Build history of the part. All positions in model axes, mm. Face numbers are marked on the shaded views. Round coordinates to 2 decimals unless told otherwise and drop trailing zeros. Order: outer loops, then holes, each group sorted by start corner. A loop starts at its lowest first (then second) coordinate and runs counter-clockwise, first axis right, second up. Notation, with made-up numbers: (76, 6) -> (132, 6) arc R36 cw to (132, 40) -> close; hole circle Ø6 at (72.25, -13). An arc over 180 degrees is marked (long way). Use a Markdown table: item, result. Add a question column.
Item 1: Pin check, flat tips, straight feed: pin 1 (3 mm diameter, centred on x = 10, y = 9, fed in from +Z); pin 2 (1.5 mm diameter, centred on y = 15, z = -1.5, fed in from +X); pin 3 (3 mm diameter, centred on x = 4.5, z = 16.5, fed in from -Y); pin 4 (6 mm diameter, centred on x = 13.5, z = 4, fed in from -Y). Stop position of each tip, or through.
Item 2: Slice it at C-C, the plane z = 8.5. Give the cut face in (x, y), plus the area to 3 significant figures.
Item 3: Probe L1, parallel to Y at x = 0.95, z = 0; L2, parallel to Y at x = 15, z = 0; L3, parallel to Y at x = 1.75, z = -17.5. List the from-to ranges inside material, lowest first.
Item 4: Slice it at A-A, the plane z = 0. Give the cut face in (x, y).
Item 5: Two-plate mould, pull along Z, no slides. Class the marked faces 1, 2 and 3: released by +Z, released by -Z, zero draft, split by the parting line, or undercut.
Item 6: Slice it at B-B, the plane y = 0. Give the cut face in (x, z).
Item 7: Slice it at D-D, the plane x = 10.5. Give the cut face in (y, z).
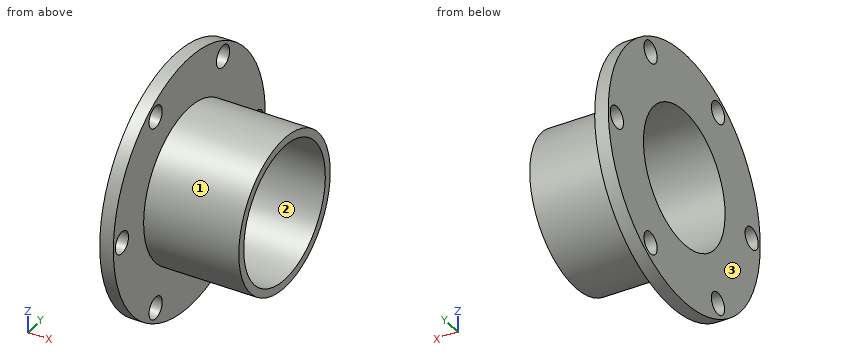
from build123d import *

# Parameters (mm, degrees)
SKETCH1_R           = 23.276074499
SKETCH1_R_2         = 2.0193
BOSS_EXTRUDE1_DEPTH = 2.5
SKETCH4_R           = 14
CUT_EXTRUDE2_DEPTH  = 30.8125
SKETCH5_R           = 14
SKETCH5_R_2         = 12.5
BOSS_EXTRUDE2_DEPTH = 20


with BuildPart() as part:
    # Sketch1 → Boss-Extrude1 (new body)
    with BuildSketch(Plane(origin=(0, 0, 0), x_dir=(0, 0, -1), z_dir=(1, 0, 0))):
        Circle(SKETCH1_R)
        with Locations((0, 20.64)):
            Circle(SKETCH1_R_2, mode=Mode.SUBTRACT)
        with Locations((17.874764334, 10.32)):
            Circle(SKETCH1_R_2, mode=Mode.SUBTRACT)
        with Locations((17.874764334, -10.32)):
            Circle(SKETCH1_R_2, mode=Mode.SUBTRACT)
        with Locations((0, -20.64)):
            Circle(SKETCH1_R_2, mode=Mode.SUBTRACT)
        with Locations((-17.874764334, -10.32)):
            Circle(SKETCH1_R_2, mode=Mode.SUBTRACT)
        with Locations((-17.874764334, 10.32)):
            Circle(SKETCH1_R_2, mode=Mode.SUBTRACT)
    extrude(amount=BOSS_EXTRUDE1_DEPTH)

    # Sketch4 → Cut-Extrude2 (cut)
    with BuildSketch(Plane.ZY):
        Circle(SKETCH4_R)
    extrude(amount=-CUT_EXTRUDE2_DEPTH, mode=Mode.SUBTRACT)

    # Sketch5 → Boss-Extrude2 (add)
    with BuildSketch(Plane(origin=(0, 0, 0), x_dir=(0, 0, -1), z_dir=(1, 0, 0))):
        Circle(SKETCH5_R)
        Circle(SKETCH5_R_2, mode=Mode.SUBTRACT)
    extrude(amount=BOSS_EXTRUDE2_DEPTH)


solid = part.part
Check sheet entries:
| question | item | result |
|---|---|---|
| 1 | pin 1 | z = 11.82 |
| 1 | pin 2 | x = 2.5 |
| 1 | pin 3 | through |
| 1 | pin 4 | y = -13.96 |
| 2 | outline | (0, -21.67) -> (2.5, -21.67) -> (2.5, -11.12) -> (20, -11.12) -> (20, -9.17) -> (0, -9.17) -> close; (0, 9.17) -> (20, 9.17) -> (20, 11.12) -> (2.5, 11.12) -> (2.5, 21.67) -> (0, 21.67) -> close |
| 2 | area | 131 mm2 |
| 3 | L1 | -23.28 to -22.66, -18.62 to -12.5, 12.5 to 18.62, 22.66 to 23.28 |
| 3 | L2 | -14 to -12.5, 12.5 to 14 |
| 3 | L3 | -15.35 to -12.3, -8.34 to 8.34, 12.3 to 15.35 |
| 4 | outline | (0, -23.28) -> (2.5, -23.28) -> (2.5, -22.66) -> (0, -22.66) -> close; (0, -18.62) -> (2.5, -18.62) -> (2.5, -14) -> (20, -14) -> (20, -12.5) -> (0, -12.5) -> close; (0, 12.5) -> (20, 12.5) -> (20, 14) -> (2.5, 14) -> (2.5, 18.62) -> (0, 18.62) -> close; (0, 22.66) -> (2.5, 22.66) -> (2.5, 23.28) -> (0, 23.28) -> close |
| 5 | face 1 | split by the parting line |
| 5 | face 2 | undercut |
| 5 | face 3 | zero draft |
| 6 | outline | (0, -23.28) -> (2.5, -23.28) -> (2.5, -14) -> (20, -14) -> (20, -12.5) -> (0, -12.5) -> close; (0, 12.5) -> (20, 12.5) -> (20, 14) -> (2.5, 14) -> (2.5, 23.28) -> (0, 23.28) -> close |
| 7 | outline | circle Ø28 at (0, 0); hole circle Ø25 at (0, 0) |
